Read the model definition and answer for the solid it produces. Units are mm, in the model's axes. A direction names the side the tool comes from. Coordinates: 2 decimals unless noted, no trailing zeros. Write each loop counter-clockwise with the first axis right and the second up, starting at its lowest first coordinate (ties: lowest second). Pieces come first, ordered by that corner, then holes.
(1) Which of the six approach directions +Z, -Z, +X, -X, +Y, -Y give full straight-line access (tool end or side, diameter ignored) to faces 4 (the flat face through (85.557, 2, -59)), 5 (the cylindrical face through (33.71, 3.01, -4.43)), 6 (the flat face through (95.613, 2, -54))?
(2) Find the intervals of material crossed by probe 1 along X at (y, z) = (3.15, -42); probe 2 along X at (y, z) = (1.7, 0); probe 3 along X at (y, z) = (1.7, -30), in increasing order.
(3) Section A-A on x = 92 is taken. Write down the section's boundary in (y, z), then the cut area to 3 significant figures.
(4) Section C-C on x = 6.5 is taken. Write down the section's boundary in (y, z), then the cut area to 3 significant figures.
(5) Section D-D on z = -23 is taken. Write down the section's boundary in (x, y).
(6) Given pin 1 (4.5 mm diameter, centred on x = 6.5, z = -15.5, fed in from -Y); pin 2 (3 mm diameter, centred on x = -92, z = 42, fed in from +Y); pin 3 (2 mm diameter, centred on x = 73.5, y = 1, fed in from -Z), each flat-ended and moving along its own axis, determine where each tip first touches the part or whether it passes through.
(7) Section B-B on z = 0 is taken. Write down the section's boundary in (x, y), then the cut area to 3 significant figures.
(8) The mould has two halves that part along X. Classify faces 1 (the flat face through (-97, 2, 48)), 2 (the flat face through (92, 2, -61.418)), 3 (the cylindrical face through (94, 2, -42)): +X half, -X half, draft (parallel to the pull), parting line (faces both ways), or undercut.
from build123d import *

# Parameters (mm, degrees)
ESQUISSE2_W             = 200
ESQUISSE2_H             = 100
ESQUISSE2_R             = 4.5
ESQUISSE2_R_2           = 2
BOSS_EXTRU_1_DEPTH      = 4
ESQUISSE3_R             = 34
ESQUISSE3_R_2           = 30
ENL_V_MAT_EXTRU_1_DEPTH = 2
ENL_V_MAT_EXTRU_2_DEPTH = 10
BOSS_EXTRU_2_DEPTH      = 4
CHANFREIN1_SIZE         = 5
CHANFREIN2_SIZE         = 2


with BuildPart() as part:
    # Esquisse2 → Boss.-Extru.1 (new body)
    with BuildSketch(Plane(origin=(0, 0, 0), x_dir=(1, 0, 0), z_dir=(0, 1, 0))):
        Rectangle(ESQUISSE2_W, ESQUISSE2_H)
        with Locations(Location((0, 0, 0), (0, 0, 270))):
            Circle(ESQUISSE2_R, mode=Mode.SUBTRACT)
        with Locations(Location((6.5, 15.5, 0), (0, 0, 270))):
            Circle(ESQUISSE2_R_2, mode=Mode.SUBTRACT)
        with Locations(Location((6.5, -15.5, 0), (0, 0, 90))):
            Circle(ESQUISSE2_R_2, mode=Mode.SUBTRACT)
        with Locations(Location((-20, 0, 0), (0, 0, 270))):
            Circle(ESQUISSE2_R_2, mode=Mode.SUBTRACT)
        with Locations(Location((92, 42, 0), (0, 0, 270))):
            Circle(ESQUISSE2_R_2, mode=Mode.SUBTRACT)
        with Locations(Location((-92, 42, 0), (0, 0, 90))):
            Circle(ESQUISSE2_R_2, mode=Mode.SUBTRACT)
        with Locations(Location((-92, -42, 0), (0, 0, 270))):
            Circle(ESQUISSE2_R_2, mode=Mode.SUBTRACT)
        with Locations(Location((92, -42, 0), (0, 0, 90))):
            Circle(ESQUISSE2_R_2, mode=Mode.SUBTRACT)
    extrude(amount=BOSS_EXTRU_1_DEPTH)

    # Esquisse3 → Enlèv. mat.-Extru.1 (cut)
    with BuildSketch(Plane(origin=(0, 4, 0), x_dir=(1, 0, 0), z_dir=(0, 1, 0))):
        with Locations(Location((0, 0, 0), (0, 0, 270))):
            Circle(ESQUISSE3_R)
        with Locations(Location((0, 0, 0), (0, 0, 270))):
            Circle(ESQUISSE3_R_2, mode=Mode.SUBTRACT)
    extrude(amount=-ENL_V_MAT_EXTRU_1_DEPTH, mode=Mode.SUBTRACT)

    # Esquisse4 → Enlèv. mat.-Extru.2 (cut)
    with BuildSketch(Plane(origin=(0, 4, 0), x_dir=(1, 0, 0), z_dir=(0, 1, 0))):
        with BuildLine():
            Line((-84.578253972, 34.018938554), (-84.578253972, -30.428285652))
            add(Edge.make_bspline(
                [(-84.578253972, -30.428285652), (-84.141978558, -34.833934515), (-79.702813843, -35.456083285)],
                knots=[0, 0, 0, 1, 1, 1], degree=2))
            Line((-79.702813843, -35.456083285), (-46.945950476, -35.456083285))
            add(Edge.make_bspline(
                [(-43.289370379, -30.428285652), (-43.697579242, -34.066767069), (-46.945950476, -35.456083285)],
                knots=[0, 0, 0, 1, 1, 1], degree=2))
            Line((-43.289370379, -30.428285652), (-43.289370379, 34.018938554))
            add(Edge.make_bspline(
                [(-46.945950476, 38.894378683), (-43.822752081, 37.558044403), (-43.289370379, 34.018938554)],
                knots=[0, 0, 0, 1, 1, 1], degree=2))
            Line((-46.945950476, 38.894378683), (-79.702813843, 38.894378683))
            add(Edge.make_bspline(
                [(-79.702813843, 38.894378683), (-84.282201555, 38.592094199), (-84.578253972, 34.018938554)],
                knots=[0, 0, 0, 1, 1, 1], degree=2))
        make_face()
        with BuildLine():
            Line((79.702813843, -35.456083285), (46.945950476, -35.456083285))
            add(Edge.make_bspline(
                [(43.289370379, -30.428285652), (43.697579242, -34.066767069), (46.945950476, -35.456083285)],
                knots=[0, 0, 0, 1, 1, 1], degree=2))
            Line((43.289370379, -30.428285652), (43.289370379, 34.018938554))
            add(Edge.make_bspline(
                [(46.945950476, 38.894378683), (43.822752081, 37.558044403), (43.289370379, 34.018938554)],
                knots=[0, 0, 0, 1, 1, 1], degree=2))
            Line((46.945950476, 38.894378683), (79.702813843, 38.894378683))
            add(Edge.make_bspline(
                [(79.702813843, 38.894378683), (84.282201555, 38.592094199), (84.578253972, 34.018938554)],
                knots=[0, 0, 0, 1, 1, 1], degree=2))
            Line((84.578253972, 34.018938554), (84.578253972, -30.428285652))
            add(Edge.make_bspline(
                [(84.578253972, -30.428285652), (84.141978558, -34.833934515), (79.702813843, -35.456083285)],
                knots=[0, 0, 0, 1, 1, 1], degree=2))
        make_face()
    extrude(amount=-ENL_V_MAT_EXTRU_2_DEPTH, mode=Mode.SUBTRACT)

    # Esquisse5 → Boss.-Extru.2 (add)
    with BuildSketch(Plane.XZ):
        Polygon((100, -50), (100, -61.418367617), (85.556933512, -61.418367617), (85.556933512, -57), (95.612528779, -57), (95.612528779, -50), align=None)
    boss_extru_2 = extrude(amount=-BOSS_EXTRU_2_DEPTH)

    # Symétrie1: Boss.-Extru.2 across plane
    add(boss_extru_2.mirror(Plane(origin=(0, 0, 0), x_dir=(0, 0, 1), z_dir=(1, 0, 0))))

    # Chanfrein1
    chanfrein1_edges = [part.edges().sort_by_distance(p)[0] for p in [
        (100, 2, 50),
        (-100, 2, 50),
    ]]
    chamfer(chanfrein1_edges, length=CHANFREIN1_SIZE)

    # Chanfrein2
    chanfrein2_edges = [part.edges().sort_by_distance(p)[0] for p in [
        (100, 2, -61.418367617),
        (-100, 2, -61.418367617),
    ]]
    chamfer(chanfrein2_edges, length=CHANFREIN2_SIZE)


solid = part.part
Response:
1. face 4: -Z, +Y, -Y
1. face 5: +Y
1. face 6: +Y, -Y
2. probe 1: x = -100 to -94, -90 to 90, 94 to 100
2. probe 2: x = -100 to -84.58, -43.29 to -22, -18 to -4.5, 4.5 to 43.29, 84.58 to 100
2. probe 3: x = -100 to -84.58, -43.29 to 43.29, 84.58 to 100
3. outline: (0, -61.42) - (4, -61.42) - (4, -57) - (0, -57) - close; (0, -50) - (4, -50) - (4, -44) - (0, -44) - close; (0, -40) - (4, -40) - (4, 40) - (0, 40) - close; (0, 44) - (4, 44) - (4, 50) - (0, 50) - close
3. area: 386 mm2
4. outline: (0, -50) - (4, -50) - (4, -33.37) - (2, -33.37) - (2, -29.29) - (4, -29.29) - (4, -17.5) - (0, -17.5) - close; (0, -13.5) - (4, -13.5) - (4, 13.5) - (0, 13.5) - close; (0, 17.5) - (4, 17.5) - (4, 29.29) - (2, 29.29) - (2, 33.37) - (4, 33.37) - (4, 50) - (0, 50) - close
4. area: 352 mm2
5. outline: (-100, 0) - (-84.58, 0) - (-84.58, 4) - (-100, 4) - close; (-43.29, 0) - (43.29, 0) - (43.29, 4) - (25.04, 4) - (25.04, 2) - (19.26, 2) - (19.26, 4) - (-19.26, 4) - (-19.26, 2) - (-25.04, 2) - (-25.04, 4) - (-43.29, 4) - close; (84.58, 0) - (100, 0) - (100, 4) - (84.58, 4) - close
6. pin 1: stops at y = 0
6. pin 2: passes through
6. pin 3: stops at z = -50
7. outline: (-100, 0) - (-84.58, 0) - (-84.58, 4) - (-100, 4) - close; (-43.29, 0) - (-22, 0) - (-22, 4) - (-30, 4) - (-30, 2) - (-34, 2) - (-34, 4) - (-43.29, 4) - close; (-18, 0) - (-4.5, 0) - (-4.5, 4) - (-18, 4) - close; (4.5, 0) - (43.29, 0) - (43.29, 4) - (34, 4) - (34, 2) - (30, 2) - (30, 4) - (4.5, 4) - close; (84.58, 0) - (100, 0) - (100, 4) - (84.58, 4) - close
7. area: 402 mm2
8. face 1: -X half
8. face 2: draft
8. face 3: undercut
